Geometry check sheet. Reference: the model listing, model coordinates, mm. Face numbers are marked on the shaded views. A direction names the side the tool comes from. Coordinates: 2 decimals unless noted, no trailing zeros. Loops run counter-clockwise (first coordinate to the right, second up) from the corner with the lowest first, then second, coordinate; pieces in that order, holes last.
from build123d import *

# Parameters (mm, degrees)
F1_DEPTH    = 63.5
F0_W        = 26.465196414
F0_H        = 19.05
F2_DEPTH    = 25.4
F3_DEPTH    = 7.9375
F5_R        = 6.35
F6_T4_ANGLE = 180


# Not quite as in the source:
# - a fillet or chamfer that OpenCascade refuses, or shapes differently, is made with other operations: its cross-section is extruded or revolved along the edge and cut away or added


with BuildPart() as f1:
    # F0 (on Front) → F1 (new body, symmetric)
    with BuildSketch(Plane.XZ):
        Polygon((-41.275, -9.525), (41.275, -9.525), (41.275, 9.525), (22.225, 9.525), (-41.275, 9.525), align=None)
    extrude(amount=F1_DEPTH, both=True)

    # F0 (on Front) → F2 (join, symmetric)
    with BuildSketch(Plane.XZ):
        with BuildLine():
            Line((22.225, 9.525), (41.275, 9.525))
            Line((41.275, 9.525), (41.275, 27.0002))
            ThreePointArc((41.275, 27.0002), (45.9246798487, 38.2255201513), (57.15, 42.8752))
            Line((57.15, 42.8752), (66.675, 42.8752))
            Line((66.675, 42.8752), (66.675, 61.9252))
            Line((66.675, 61.9252), (57.15, 61.9252))
            add(Edge.make_bspline(
                [(56.9072220114, 61.9243561652), (56.9881728551, 61.9246965832), (57.0690989666, 61.9249778596), (57.15, 61.9252)],
                knots=[111.2968717992, 111.2968717992, 111.2968717992, 111.2968717992, 111.5045361635, 111.5045361635, 111.5045361635, 111.5045361635], degree=3))
            ThreePointArc((56.9072220114, 61.9243561652), (32.3686093383, 51.6099196626), (22.225, 27.0002))
            Line((22.225, 27.0002), (22.225, 9.525))
        make_face()
        with Locations((79.907598207, 52.4002)):
            Rectangle(F0_W, F0_H)
    extrude(amount=F2_DEPTH, both=True)

    # F0 (on Front) → F3 (join, symmetric)
    with BuildSketch(Plane.XZ):
        with BuildLine():
            add(Edge.make_bspline(
                [(-41.275, 9.525), (-36.9673291938, 44.5717190185), (13.5219464317, 61.7419104925), (56.9072220114, 61.9243561652)],
                knots=[0, 0, 0, 0, 111.2968717992, 111.2968717992, 111.2968717992, 111.2968717992], degree=3))
            Line((-41.275, 9.525), (22.225, 9.525))
            Line((22.225, 9.525), (22.225, 27.0002))
            ThreePointArc((22.225, 27.0002), (32.3686093383, 51.6099196626), (56.9072220114, 61.9243561652))
        make_face()
    extrude(amount=F3_DEPTH, both=True)

    # F0 (on Front) → F4 (revolve)
    with BuildSketch(Plane.XZ):
        Polygon((93.140196414, 61.9252), (93.140196414, 42.8752), (93.140196414, 38.1), (117.475, 38.1), (117.475, 66.675), (93.140196414, 66.675), align=None)
    revolve(axis=Axis((93.140196414, 0, 52.3875), (0, 0, -1)))

    # F5
    f5_edges = [f1.edges().sort_by_distance(p)[0] for p in [
        (-41.275, 63.5, 0),
        (-41.275, -63.5, 0),
        (41.275, -63.5, 0),
        (41.275, 63.5, 0),
    ]]
    fillet(f5_edges, radius=F5_R)

    # F6: fillet of radius 10.16 on 1 edges, made by hand


with BuildPart() as f6_tool2:
    # F6_s3 → F6_t4 (revolve)
    with BuildSketch(Plane.YZ.offset(93.140196414)):
        with BuildLine():
            ThreePointArc((32.9345324166, 61.9252), (28.0224061967, 63.1915721688), (24.334803586, 66.675))
            Line((24.334803586, 66.675), (24.334803586, 61.9252))
            Line((24.334803586, 61.9252), (32.9345324166, 61.9252))
        make_face()
    revolve(axis=Axis((93.140196414, 0, 61.9252), (0, 0, 1)), revolution_arc=F6_T4_ANGLE)

    split(bisect_by=Plane.XZ.offset(-25.4), keep=Keep.TOP)

    split(bisect_by=Plane.XZ.offset(25.4), keep=Keep.BOTTOM)


with BuildPart() as f1_1:
    add(f1.part)

    # F6_t1: union F6_tool2
    add(f6_tool2.part)


solid = f1_1.part
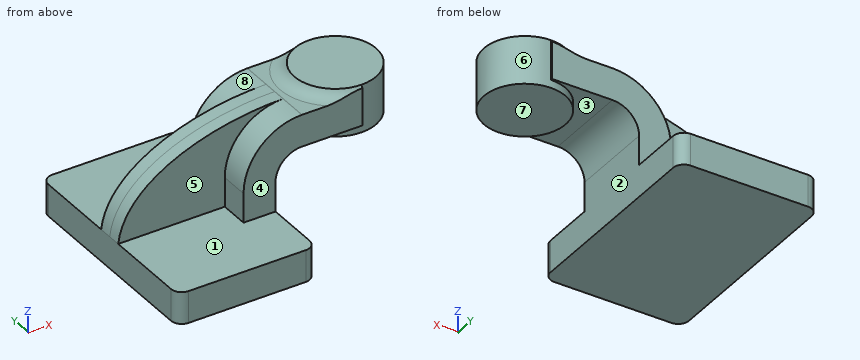
(1) Sectioned sample at B-B on y = 35.5. Record the cut outline in (x, z) (3 decimals), and give its area (3 significant figures).
Findings:
outline: (-41.275, -9.525) - (41.275, -9.525) - (41.275, 9.525) - (-41.275, 9.525) - close
area: 1,570 mm2
(2) Draft check along X on the marked faces 1, 2 and 3. Enter one of: +X half, -X half, draft (parallel to the pull), parting line (faces both ways), or undercut.
Findings:
face 1: draft
face 2: +X half
face 3: undercut
(3) Sectioned sample at A-A on z = 2.5. Record the cut outline in (x, y) (3 decimals), and give its area (3 significant figures).
Findings:
outline: (-41.275, -57.15) arc R6.35 ccw to (-34.925, -63.5) - (34.925, -63.5) arc R6.35 ccw to (41.275, -57.15) - (41.275, 57.15) arc R6.35 ccw to (34.925, 63.5) - (-34.925, 63.5) arc R6.35 ccw to (-41.275, 57.15) - close
area: 10,400 mm2
(4) Scan lines: L1, parallel to Y at x = 81, z = 48; L2, parallel to X at y = -40, z = 4 (3 decimals); L3, parallel to Z at x = -33.5, y = 9.5 (3 decimals). Record each from-to range of solid material in increasing order.
Findings:
L1: y = -25.4 to 25.4
L2: x = -41.275 to 41.275
L3: z = -9.525 to 9.525
(5) Gauge pin test, flat ends, axial feed: pin 1 Ø8.5 at (y, z) = (-18, 14) entering from -X (3 decimals); pin 2 Ø0.5 at (y, z) = (-25, 50.5) entering from +X; pin 3 Ø5 at (x, z) = (-16.5, 36) entering from +Y. Record the tip position at first contact, or that the pin passes through.
Findings:
pin 1: stops at x = 22.225
pin 2: stops at x = 93.14
pin 3: stops at y = 7.94
(6) Access from +Z, -Z, +X, -X, +Y, -Y to the whole of each face (thin tool, end or side, straight path). Record for the marked faces 4, 5, 6, 7 and 8.
Findings:
face 4: +Z, +X, -X, -Y
face 5: +Z, -X, -Y
face 6: -Z
face 7: -Z, +X, +Y, -Y
face 8: +Z, -X, +Y
